Design review of the part built by this model. Coordinates are the model's own, in mm. A direction names the side the tool comes from. Coordinates: 2 decimals unless noted, no trailing zeros. Order: outer loops, then holes, each group sorted by start corner. A loop starts at its lowest first (then second) coordinate and runs counter-clockwise, first axis right, second up. Notation, with made-up numbers: (72.25, 48) -> (98.25, 48) arc R35 ccw to (98.25, 80) -> close; hole circle Ø5 at (-5.75, -34). An arc over 180 degrees is marked (long way). Write item = value, one per line.
```python
from build123d import *

# Parameters (mm, degrees)
BOX_W             = 10
BOX_H             = 1
BOX_DEPTH         = 14
CYLINDER002_R     = 3.75
CYLINDER002_DEPTH = 14
CYLINDER001_R     = 8
CYLINDER001_DEPTH = 1.5
CYLINDER_R        = 6
CYLINDER_DEPTH    = 11.5


with BuildPart() as opening:
    # Box → Box (new body)
    with BuildSketch(Plane(origin=(0, -0.5, -1), x_dir=(1, 0, 0), z_dir=(0, 0, 1))):
        with Locations((5, 0.5)):
            Rectangle(BOX_W, BOX_H)
    extrude(amount=BOX_DEPTH)


with BuildPart() as inner:
    # Cylinder002 → Cylinder002 (new body)
    with BuildSketch(Plane.XY.offset(-1)):
        Circle(CYLINDER002_R)
    extrude(amount=CYLINDER002_DEPTH)


with BuildPart() as base:
    # Cylinder001 → Cylinder001 (new body)
    with BuildSketch(Plane.XY):
        Circle(CYLINDER001_R)
    extrude(amount=CYLINDER001_DEPTH)


with BuildPart() as gap:
    # Cylinder → Cylinder (new body)
    with BuildSketch(Plane.XY):
        Circle(CYLINDER_R)
    extrude(amount=CYLINDER_DEPTH)

    # Fusion: union base
    add(base.part)

    # Cut: cut inner
    add(inner.part, mode=Mode.SUBTRACT)

    # Cut001: cut opening
    add(opening.part, mode=Mode.SUBTRACT)


solid = gap.part
```
(1) For L1, parallel to Y at x = 0, z = 9; L2, parallel to Z at x = -2.5, y = -6; L3, parallel to X at y = 0, z = 6, list the stretches that pass through material, from the lowest coordinate up.
Report:
L1 = -6 to -3.75, 3.75 to 6
L2 = 0 to 1.5
L3 = -6 to -3.75
(2) For faces 5 (the flat face through (-1.9, -3.44, 0)), 6 (the flat face through (-3, 5.4, 1.5)), 7 (the flat face through (5, 0.5, 6)), list the 3-axis set-ups (+Z, -Z, +X, -X, +Y, -Y) from which the entire face can be reached by the end or side of a thin tool; tool diameter is ignored.
Report:
face_5 = -Z, +X, -X, +Y, -Y
face_6 = +Z
face_7 = +Z, -Z, +X
(3) We need section C-C (x = 6.5). Write out the cut boundary in (y, z).
Report:
outline = (-4.66, 0) -> (-0.5, 0) -> (-0.5, 1.5) -> (-4.66, 1.5) -> close; (0.5, 0) -> (4.66, 0) -> (4.66, 1.5) -> (0.5, 1.5) -> close
(4) We need section D-D (y = 0). Write out the cut boundary in (x, z), and give its area (3 significant figures).
Report:
outline = (-8, 0) -> (-3.75, 0) -> (-3.75, 11.5) -> (-6, 11.5) -> (-6, 1.5) -> (-8, 1.5) -> close
area = 28.9 mm²
(5) We need section A-A (x = 0). Write out the cut boundary in (y, z), and give its area (4 significant figures).
Report:
outline = (-8, 0) -> (-3.75, 0) -> (-3.75, 11.5) -> (-6, 11.5) -> (-6, 1.5) -> (-8, 1.5) -> close; (3.75, 0) -> (8, 0) -> (8, 1.5) -> (6, 1.5) -> (6, 11.5) -> (3.75, 11.5) -> close
area = 57.75 mm²
(6) Insertion check: pin 1 (4.5 mm diameter, centred on x = 0, y = 0, fed in from -Z); pin 2 (2 mm diameter, centred on x = -5.5, y = 4.5, fed in from +Z); pin 3 (1 mm diameter, centred on y = -2, z = 3, fed in from -X); pin 4 (1.3 mm diameter, centred on x = 5, z = 6, fed in from +Y). Each pin has a flat end and moves straight along its axis. Give the tip position at first contact, or say it passes through.
Report:
pin_1 = through
pin_2 = 1.5
pin_3 = -5.81
pin_4 = 4.13
(7) We need section B-B (y = 3). Write out the cut boundary in (x, z), and give its area (3 significant figures).
Report:
outline = (-7.42, 0) -> (-2.25, 0) -> (-2.25, 11.5) -> (-5.2, 11.5) -> (-5.2, 1.5) -> (-7.42, 1.5) -> close; (2.25, 0) -> (7.42, 0) -> (7.42, 1.5) -> (5.2, 1.5) -> (5.2, 11.5) -> (2.25, 11.5) -> close
area = 74.4 mm²
(8) The part is to be moulded in two halves that separate along Y. For faces 1 (the flat face through (-3, -3, 11.5)), 2 (the flat face through (5, -0.5, 6)), 3 (the cylindrical face through (-3.747, 0.158, 5.67)), 4 (the cylindrical face through (-8, 0, 1)), say which applies: released by +Y, released by -Y, zero draft, split by the parting line, or undercut.
Report:
face_1 = zero draft
face_2 = undercut
face_3 = undercut
face_4 = split by the parting line
